```python
from build123d import *

# Parameters (mm, degrees)
SKETCH1_W           = 44.45
SKETCH1_H           = 25.4
SKETCH1_R           = 1.524
BOSS_EXTRUDE1_DEPTH = 2.54
FILLET1_R           = 2.54


with BuildPart() as part:
    # Sketch1 → Boss-Extrude1 (new body)
    with BuildSketch(Plane.XY):
        with Locations((17.145, -28.589614644)):
            Rectangle(SKETCH1_W, SKETCH1_H)
        with Locations((12.482257686, -28.589614644)):
            Circle(SKETCH1_R, mode=Mode.SUBTRACT)
        with Locations((28.357257686, -28.589614644)):
            Circle(SKETCH1_R, mode=Mode.SUBTRACT)
        with Locations((12.482257686, -19.699614644)):
            Circle(SKETCH1_R, mode=Mode.SUBTRACT)
        with Locations((28.357257686, -19.699614644)):
            Circle(SKETCH1_R, mode=Mode.SUBTRACT)
        with Locations((12.482257686, -37.479614644)):
            Circle(SKETCH1_R, mode=Mode.SUBTRACT)
        with Locations((28.357257686, -37.479614644)):
            Circle(SKETCH1_R, mode=Mode.SUBTRACT)
        with Locations((-2.231491516, -28.589614644)):
            Circle(SKETCH1_R, mode=Mode.SUBTRACT)
        with Locations((35.868508484, -28.589614644)):
            Circle(SKETCH1_R, mode=Mode.SUBTRACT)
    extrude(amount=BOSS_EXTRUDE1_DEPTH)

    # Fillet1
    fillet1_edges = [part.edges().sort_by_distance(p)[0] for p in [
        (-5.08, -15.889614644, 1.27),
        (39.37, -15.889614644, 1.27),
        (39.37, -41.289614644, 1.27),
        (-5.08, -41.289614644, 1.27),
    ]]
    fillet(fillet1_edges, radius=FILLET1_R)


solid = part.part
```
CAD build for the part. Positions are in the model's coordinates, mm. Coordinates: 2 decimals unless noted, no trailing zeros. Write each loop counter-clockwise with the first axis right and the second up, starting at its lowest first coordinate (ties: lowest second). Pieces come first, ordered by that corner, then holes. Notation, with made-up numbers: (23.25, -26.5) -> (36.25, -26.5) arc R26 cw to (36.25, 9.5) -> close; hole circle Ø5 at (12.5, -9). An arc over 180 degrees is marked (long way). Use CSV: the item, a comma, the result in double quotes. Start each with the question number.
Item 1: Band-saw the part on A-A, the plane x = 35. Write the cut outline in (y, z).
Item 2: Two-plate mould, pull along Y, no slides. Class faces 1 (the flat face through (17, -28, 0)), 2 (the cylindrical face through (38.606, -16.614, 1.288)), 3 (the cylindrical face through (12.28, -27.08, 1.25)), 4 (the cylindrical face through (29.06, -38.83, 1.25)): +Y half, -Y half, draft (parallel to the pull), parting line (faces both ways), or undercut.
Item 3: Band-saw the part on B-B, the plane z = 1.55. Give the number of separate pieces and of enclosed holes in the cut face, plus the area to 3 significant figures.
Item 4: Drop a flat-ended pin along its axis: P1, Ø1.5, axis at x = 15.5, y = -36, coming from the -Z side. Give the stop position or say it passes through.
Item 5: Wall check: probe 1 along X at (y, z) = (-19.25, 0.45); probe 2 along X at (y, z) = (-29.75, 2.1); probe 3 along Y at (x, z) = (29.5, 2.25). Give the ranges that are in metal, low to high.
Response values:
1,outline,"(-41.29, 0) -> (-29.84, 0) -> (-29.84, 2.54) -> (-41.29, 2.54) -> close; (-27.34, 0) -> (-15.89, 0) -> (-15.89, 2.54) -> (-27.34, 2.54) -> close"
2,face 1,"draft"
2,face 2,"+Y half"
2,face 3,"undercut"
2,face 4,"undercut"
3,separate pieces,"1"
3,enclosed holes,"8"
3,area,"1,070 mm2"
4,P1,"stops at z = 0"
5,probe 1,"x = -5.08 to 11.03, 13.94 to 26.9, 29.81 to 39.37"
5,probe 2,"x = -5.08 to -3.22, -1.24 to 11.49, 13.47 to 27.37, 29.35 to 34.88, 36.86 to 39.37"
5,probe 3,"y = -41.29 to -38.49, -36.47 to -29.6, -27.58 to -20.71, -18.69 to -15.89"
